Verification items for the finished model (mm, model axes). A direction names the side the tool comes from. Round coordinates to 2 decimals unless told otherwise and drop trailing zeros. Write each loop counter-clockwise with the first axis right and the second up, starting at its lowest first coordinate (ties: lowest second). Pieces come first, ordered by that corner, then holes. Notation, with made-up numbers: M 66.5,36 L 94.5,36 A32 ccw 94.5,62 Z; hole C 42,48.5 d10. An arc over 180 degrees is marked long. One line per question, with ' | ' between items.
from build123d import *

# Parameters (mm, degrees)
SKETCH1_R           = 8
BOSS_EXTRUDE1_DEPTH = 10
SKETCH1_3_R         = 8
BOSS_EXTRUDE2_DEPTH = 4


with BuildPart() as part:
    # Sketch1 → Boss-Extrude1 (new, symmetric)
    # profile 1 of 10: a face of its own
    with BuildSketch(Plane.XY):
        with BuildLine():
            Line((28.701257427, 69.290964938), (22.961005942, 55.432771951))
            ThreePointArc((22.961005942, 55.432771951), (42.426406871, 42.426406871), (55.432771951, 22.961005942))
            Line((55.432771951, 22.961005942), (69.290964938, 28.701257427))
            ThreePointArc((69.290964938, 28.701257427), (53.033008589, 53.033008589), (28.701257427, 69.290964938))
        make_face()
    # profile 2 of 10: a face of its own
    with BuildSketch(Plane.XY):
        with BuildLine():
            Line((22.961005942, 55.432771951), (9.567085809, 23.096988313))
            ThreePointArc((9.567085809, 23.096988313), (17.67766953, 17.67766953), (23.096988313, 9.567085809))
            Line((23.096988313, 9.567085809), (55.432771951, 22.961005942))
            ThreePointArc((55.432771951, 22.961005942), (42.426406871, 42.426406871), (22.961005942, 55.432771951))
        make_face()
    # profile 3 of 10: a face of its own
    with BuildSketch(Plane.XY):
        with BuildLine():
            Line((55.432771951, -22.961005942), (23.096988313, -9.567085809))
            ThreePointArc((23.096988313, -9.567085809), (17.67766953, -17.67766953), (9.567085809, -23.096988313))
            Line((9.567085809, -23.096988313), (22.961005942, -55.432771951))
            ThreePointArc((22.961005942, -55.432771951), (42.426406871, -42.426406871), (55.432771951, -22.961005942))
        make_face()
    # profile 4 of 10: a face of its own
    with BuildSketch(Plane.XY):
        with BuildLine():
            Line((55.432771951, 22.961005942), (23.096988313, 9.567085809))
            ThreePointArc((23.096988313, 9.567085809), (24.51963201, 4.87725805), (25, 0))
            ThreePointArc((25, 0), (24.51963201, -4.87725805), (23.096988313, -9.567085809))
            Line((23.096988313, -9.567085809), (55.432771951, -22.961005942))
            ThreePointArc((55.432771951, -22.961005942), (58.847116824, -11.705419321), (60, 0))
            ThreePointArc((60, 0), (58.847116824, 11.705419321), (55.432771951, 22.961005942))
        make_face()
        with Locations((40, 0)):
            Circle(SKETCH1_R, mode=Mode.SUBTRACT)
    # profile 5 of 10: a face of its own
    with BuildSketch(Plane.XY):
        with BuildLine():
            Line((69.290964938, -28.701257427), (55.432771951, -22.961005942))
            ThreePointArc((55.432771951, -22.961005942), (42.426406871, -42.426406871), (22.961005942, -55.432771951))
            Line((22.961005942, -55.432771951), (28.701257427, -69.290964938))
            ThreePointArc((28.701257427, -69.290964938), (53.033008589, -53.033008589), (69.290964938, -28.701257427))
        make_face()
    # profile 6 of 10: a face of its own
    with BuildSketch(Plane.XY):
        with BuildLine():
            ThreePointArc((-55.432771951, 22.961005942), (-42.426406871, 42.426406871), (-22.961005942, 55.432771951))
            Line((-22.961005942, 55.432771951), (-28.701257427, 69.290964938))
            ThreePointArc((-28.701257427, 69.290964938), (-53.033008589, 53.033008589), (-69.290964938, 28.701257427))
            Line((-69.290964938, 28.701257427), (-55.432771951, 22.961005942))
        make_face()
    # profile 7 of 10: a face of its own
    with BuildSketch(Plane.XY):
        with BuildLine():
            ThreePointArc((-23.096988313, 9.567085809), (-17.67766953, 17.67766953), (-9.567085809, 23.096988313))
            Line((-9.567085809, 23.096988313), (-22.961005942, 55.432771951))
            ThreePointArc((-22.961005942, 55.432771951), (-42.426406871, 42.426406871), (-55.432771951, 22.961005942))
            Line((-55.432771951, 22.961005942), (-23.096988313, 9.567085809))
        make_face()
    # profile 8 of 10: a face of its own
    with BuildSketch(Plane.XY):
        with BuildLine():
            Line((-55.432771951, -22.961005942), (-23.096988313, -9.567085809))
            ThreePointArc((-23.096988313, -9.567085809), (-25, 0), (-23.096988313, 9.567085809))
            Line((-23.096988313, 9.567085809), (-55.432771951, 22.961005942))
            ThreePointArc((-55.432771951, 22.961005942), (-60, 0), (-55.432771951, -22.961005942))
        make_face()
        with Locations((-40, 0)):
            Circle(SKETCH1_R, mode=Mode.SUBTRACT)
    # profile 9 of 10: a face of its own
    with BuildSketch(Plane.XY):
        with BuildLine():
            ThreePointArc((-22.961005942, -55.432771951), (-42.426406871, -42.426406871), (-55.432771951, -22.961005942))
            Line((-55.432771951, -22.961005942), (-69.290964938, -28.701257427))
            ThreePointArc((-69.290964938, -28.701257427), (-53.033008589, -53.033008589), (-28.701257427, -69.290964938))
            Line((-28.701257427, -69.290964938), (-22.961005942, -55.432771951))
        make_face()
    # profile 10 of 10: a face of its own
    with BuildSketch(Plane.XY):
        with BuildLine():
            ThreePointArc((-9.567085809, -23.096988313), (-17.67766953, -17.67766953), (-23.096988313, -9.567085809))
            Line((-23.096988313, -9.567085809), (-55.432771951, -22.961005942))
            ThreePointArc((-55.432771951, -22.961005942), (-42.426406871, -42.426406871), (-22.961005942, -55.432771951))
            Line((-22.961005942, -55.432771951), (-9.567085809, -23.096988313))
        make_face()
    extrude(amount=BOSS_EXTRUDE1_DEPTH, both=True)

    # Sketch1_3 → Boss-Extrude2 (add, symmetric)
    # profile 1 of 10: a face of its own
    with BuildSketch(Plane.XY):
        with BuildLine():
            ThreePointArc((-9.567085809, 23.096988313), (0, 25), (9.567085809, 23.096988313))
            Line((9.567085809, 23.096988313), (22.961005942, 55.432771951))
            ThreePointArc((22.961005942, 55.432771951), (0, 60), (-22.961005942, 55.432771951))
            Line((-22.961005942, 55.432771951), (-9.567085809, 23.096988313))
        make_face()
        with Locations((0, 40)):
            Circle(SKETCH1_3_R, mode=Mode.SUBTRACT)
    # profile 2 of 10: a face of its own
    with BuildSketch(Plane.XY):
        with BuildLine():
            Line((22.961005942, -55.432771951), (9.567085809, -23.096988313))
            ThreePointArc((9.567085809, -23.096988313), (0, -25), (-9.567085809, -23.096988313))
            Line((-9.567085809, -23.096988313), (-22.961005942, -55.432771951))
            ThreePointArc((-22.961005942, -55.432771951), (0, -60), (22.961005942, -55.432771951))
        make_face()
        with Locations((0, -40)):
            Circle(SKETCH1_3_R, mode=Mode.SUBTRACT)
    # profile 3 of 10: a face of its own
    with BuildSketch(Plane.XY):
        with BuildLine():
            Line((-23.096988313, -9.567085809), (-18.47759065, -7.653668647))
            ThreePointArc((-18.47759065, -7.653668647), (-20, 0), (-18.47759065, 7.653668647))
            Line((-18.47759065, 7.653668647), (-23.096988313, 9.567085809))
            ThreePointArc((-23.096988313, 9.567085809), (-25, 0), (-23.096988313, -9.567085809))
        make_face()
    # profile 4 of 10: a face of its own
    with BuildSketch(Plane.XY):
        with BuildLine():
            ThreePointArc((-7.653668647, -18.47759065), (-14.142135624, -14.142135624), (-18.47759065, -7.653668647))
            Line((-18.47759065, -7.653668647), (-23.096988313, -9.567085809))
            ThreePointArc((-23.096988313, -9.567085809), (-17.67766953, -17.67766953), (-9.567085809, -23.096988313))
            Line((-9.567085809, -23.096988313), (-7.653668647, -18.47759065))
        make_face()
    # profile 5 of 10: a face of its own
    with BuildSketch(Plane.XY):
        with BuildLine():
            Line((9.567085809, -23.096988313), (7.653668647, -18.47759065))
            ThreePointArc((7.653668647, -18.47759065), (0, -20), (-7.653668647, -18.47759065))
            Line((-7.653668647, -18.47759065), (-9.567085809, -23.096988313))
            ThreePointArc((-9.567085809, -23.096988313), (0, -25), (9.567085809, -23.096988313))
        make_face()
    # profile 6 of 10: a face of its own
    with BuildSketch(Plane.XY):
        with BuildLine():
            Line((23.096988313, -9.567085809), (18.47759065, -7.653668647))
            ThreePointArc((18.47759065, -7.653668647), (14.142135624, -14.142135624), (7.653668647, -18.47759065))
            Line((7.653668647, -18.47759065), (9.567085809, -23.096988313))
            ThreePointArc((9.567085809, -23.096988313), (17.67766953, -17.67766953), (23.096988313, -9.567085809))
        make_face()
    # profile 7 of 10: a face of its own
    with BuildSketch(Plane.XY):
        with BuildLine():
            Line((23.096988313, 9.567085809), (18.47759065, 7.653668647))
            ThreePointArc((18.47759065, 7.653668647), (19.615705608, 3.90180644), (20, 0))
            ThreePointArc((20, 0), (19.615705608, -3.90180644), (18.47759065, -7.653668647))
            Line((18.47759065, -7.653668647), (23.096988313, -9.567085809))
            ThreePointArc((23.096988313, -9.567085809), (24.51963201, -4.87725805), (25, 0))
            ThreePointArc((25, 0), (24.51963201, 4.87725805), (23.096988313, 9.567085809))
        make_face()
    # profile 8 of 10: a face of its own
    with BuildSketch(Plane.XY):
        with BuildLine():
            Line((9.567085809, 23.096988313), (7.653668647, 18.47759065))
            ThreePointArc((7.653668647, 18.47759065), (14.142135624, 14.142135624), (18.47759065, 7.653668647))
            Line((18.47759065, 7.653668647), (23.096988313, 9.567085809))
            ThreePointArc((23.096988313, 9.567085809), (17.67766953, 17.67766953), (9.567085809, 23.096988313))
        make_face()
    # profile 9 of 10: a face of its own
    with BuildSketch(Plane.XY):
        with BuildLine():
            ThreePointArc((-7.653668647, 18.47759065), (0, 20), (7.653668647, 18.47759065))
            Line((7.653668647, 18.47759065), (9.567085809, 23.096988313))
            ThreePointArc((9.567085809, 23.096988313), (0, 25), (-9.567085809, 23.096988313))
            Line((-9.567085809, 23.096988313), (-7.653668647, 18.47759065))
        make_face()
    # profile 10 of 10: a face of its own
    with BuildSketch(Plane.XY):
        with BuildLine():
            ThreePointArc((-18.47759065, 7.653668647), (-14.142135624, 14.142135624), (-7.653668647, 18.47759065))
            Line((-7.653668647, 18.47759065), (-9.567085809, 23.096988313))
            ThreePointArc((-9.567085809, 23.096988313), (-17.67766953, 17.67766953), (-23.096988313, 9.567085809))
            Line((-23.096988313, 9.567085809), (-18.47759065, 7.653668647))
        make_face()
    extrude(amount=BOSS_EXTRUDE2_DEPTH, both=True)


solid = part.part
1. Section check C-C, the plane y = 14. Record the cut outline in (x, z), then the cut area to 3 significant figures.
Results:
outline: M -58.34,-10 L -20.71,-10 L -20.71,-4 L -14.28,-4 L -14.28,4 L -20.71,4 L -20.71,10 L -58.34,10 Z; M 14.28,-4 L 20.71,-4 L 20.71,-10 L 58.34,-10 L 58.34,10 L 20.71,10 L 20.71,4 L 14.28,4 Z | area: 1,610 mm2
2. Thickness scan on line 1 (Y direction, x = 0, z = 2.05); line 2 (Z direction, x = 16, y = 45); line 3 (Y direction, x = -45.5, z = 9.25). Record the ranges inside material, lowest first.
Results:
line 1: y = -60 to -48, -32 to -20, 20 to 32, 48 to 60 | line 2: z = -4 to 4 | line 3: y = -59.62 to -5.81, 5.81 to 59.62
3. Section check B-B, the plane x = 0. Record the cut outline in (y, z), then the cut area to 3 significant figures.
Results:
outline: M -60,-4 L -48,-4 L -48,4 L -60,4 Z; M -32,-4 L -20,-4 L -20,4 L -32,4 Z; M 20,-4 L 32,-4 L 32,4 L 20,4 Z; M 48,-4 L 60,-4 L 60,4 L 48,4 Z | area: 384 mm2
4. Tool access check on faces 4 (the face through (-46.349, -4.868, -0.14)), 5 (the face through (-62.26, -25.79, -0.14)), 6 (the face through (-53.324, -52.741, 0.14)), 7 (the face through (16, 14, -4)), 8 (the face through (-25, 0, 7)). Record the directions out of +Z, -Z, +X, -X, +Y, -Y that give a thin tool (end or side, any length) a straight path to the whole face; none if there is none.
Results:
face 4: +Z, -Z | face 5: +Z, -Z, -X | face 6: +Z, -Z, -X, -Y | face 7: -Z | face 8: +Z
5. Go/stop test with flat-tipped pins: P1, Ø8, axis at x = 10.5, z = 7, coming from the +Y side; P2, Ø5, axis at x = 19, z = -5, coming from the +Y side; P3, Ø6, axis at y = 2.5, z = 5, coming from the -X side. Record where each tip stops, or that it passes through.
Results:
P1: stops at y = 59.48 | P2: stops at y = 57.63 | P3: stops at x = -60
6. Mould release check, pull along Y, two halves, no side actions. Record for faces 1 (the face through (62.26, 25.79, -0.14)), 2 (the face through (53.324, 52.741, -0.14)), 3 (the face through (-27, 1, 10)): pulls with the +Y half, pulls with the -Y half, needs draft (parallel to the pull), parting line crosses it, or undercut.
Results:
face 1: undercut | face 2: pulls with the +Y half | face 3: needs draft
7. Section check D-D, the plane x = -16. Record the cut outline in (y, z).
Results:
outline: M -57.83,-4 L -38.63,-4 L -38.63,-10 L -19.21,-10 L -19.21,-4 L -12,-4 L -12,4 L -19.21,4 L -19.21,10 L -38.63,10 L -38.63,4 L -57.83,4 Z; M 12,-4 L 19.21,-4 L 19.21,-10 L 38.63,-10 L 38.63,-4 L 57.83,-4 L 57.83,4 L 38.63,4 L 38.63,10 L 19.21,10 L 19.21,4 L 12,4 Z
8. Section check A-A, the plane z = -6.5. Record the cut outline in (x, y).
Results:
outline: M -69.29,-28.7 A75 ccw -28.7,-69.29 L -9.57,-23.1 A25 cw -9.57,23.1 L -28.7,69.29 A75 ccw -69.29,28.7 L -55.43,22.96 A60 ccw -55.43,-22.96 Z; M 9.57,-23.1 L 28.7,-69.29 A75 ccw 69.29,-28.7 L 55.43,-22.96 A60 ccw 55.43,22.96 L 69.29,28.7 A75 ccw 28.7,69.29 L 9.57,23.1 A25 cw Z; hole C -40,0 d16; hole C 40,0 d16
